Verification items for the finished model (mm, model axes). Face numbers are marked on the shaded views. Coordinates: 2 decimals unless noted, no trailing zeros. Order: outer loops, then holes, each group sorted by start corner. A loop starts at its lowest first (then second) coordinate and runs counter-clockwise, first axis right, second up. Notation, with made-up numbers: (23, 62) -> (62, 62) arc R15 ccw to (62, 68) -> close; hole circle Ø2 at (-16.75, -13). An arc over 180 degrees is marked (long way). Write each question's results on one line, items separated by ' | '. Start each with the question number.
(1) Go/stop test with flat-tipped pins: pin 1 (6 mm diameter, centred on y = 1.5, z = 2, fed in from -X); pin 2 (0.8 mm diameter, centred on x = 4.5, z = -3, fed in from -Y); pin 3 (0.8 mm diameter, centred on x = 2.5, z = -3, fed in from +Y). Record where each tip stops, or that it passes through.
(2) Cross-section at C-C on x = 0.8. Enter the section's corners in (y, z), and give its area (3 significant figures).
(3) Thickness scan on probe 1 along Y at (x, z) = (3.1, 0); probe 2 along X at (y, z) = (0, -2.75); probe 3 along Z at (x, y) = (1.8, 0). Record the ranges inside material, lowest first. Write a range as [from, to].
(4) Cross-section at A-A on y = 0. Enter the section's corners in (x, z).
(5) Cross-section at B-B on z = 0. Enter the section's corners in (x, y), and give its area (3 significant figures).
(6) Cross-section at D-D on z = 2.25. Enter the section's corners in (x, y), and give its area (3 significant figures).
(7) Draft check along Y on the marked faces 1, 2 and 3. Enter one of: +Y half, -Y half, draft (parallel to the pull), parting line (faces both ways), or undercut.
```python
from build123d import *

# Parameters (mm, degrees)
F0_W     = 15
F0_H     = 15
F1_DEPTH = 1
F2_R     = 3.5
F3_DEPTH = 5
F4_R     = 2.55
F5_DEPTH = 25
F6_W     = 5.5
F6_H     = 1
F7_DEPTH = 7


with BuildPart() as f1:
    # F0 (on Right) → F1 (new body)
    with BuildSketch(Plane.YZ):
        Rectangle(F0_W, F0_H)
    extrude(amount=F1_DEPTH)

    # F2 (on face) → F3 (join)
    with BuildSketch(Plane.YZ.offset(1)):
        Circle(F2_R)
    extrude(amount=F3_DEPTH)

    # F4 (on face) → F5 (cut)
    with BuildSketch(Plane.YZ.offset(6)):
        Circle(F4_R)
    extrude(amount=-F5_DEPTH, mode=Mode.SUBTRACT)

    # F6 (on face) → F7 (cut)
    with BuildSketch(Plane(origin=(0, 0, -7.5), x_dir=(1, 0, 0), z_dir=(0, 0, -1))):
        with Locations((3.75, 0)):
            Rectangle(F6_W, F6_H)
    extrude(amount=-F7_DEPTH, mode=Mode.SUBTRACT)


solid = f1.part
```
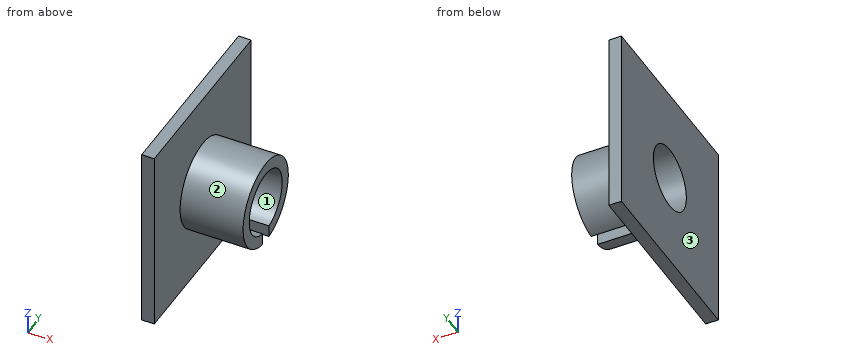
Results are:
1) pin 1: stops at x = 0 | pin 2: stops at y = -2.34 | pin 3: stops at y = 2.34
2) outline: (-7.5, -7.5) -> (7.5, -7.5) -> (7.5, 7.5) -> (-7.5, 7.5) -> close; hole circle Ø5.1 at (0, 0) | area: 205 mm2
3) probe 1: y = [-3.5, -2.55], [2.55, 3.5] | probe 2: x = [0, 1] | probe 3: z = [2.55, 3.5]
4) outline: (0, -7.5) -> (1, -7.5) -> (1, -2.55) -> (0, -2.55) -> close; (0, 2.55) -> (6, 2.55) -> (6, 3.5) -> (1, 3.5) -> (1, 7.5) -> (0, 7.5) -> close
5) outline: (0, -7.5) -> (1, -7.5) -> (1, -3.5) -> (6, -3.5) -> (6, -2.55) -> (0, -2.55) -> close; (0, 2.55) -> (6, 2.55) -> (6, 3.5) -> (1, 3.5) -> (1, 7.5) -> (0, 7.5) -> close | area: 19.4 mm2
6) outline: (0, -7.5) -> (1, -7.5) -> (1, -2.68) -> (6, -2.68) -> (6, -1.2) -> (0, -1.2) -> close; (0, 1.2) -> (6, 1.2) -> (6, 2.68) -> (1, 2.68) -> (1, 7.5) -> (0, 7.5) -> close | area: 27.4 mm2
7) face 1: undercut | face 2: parting line | face 3: draft
